```python
from build123d import *

# Parameters (mm, degrees)
BOSS_EXTRUDE1_DEPTH     = 21
SKETCH5_W               = 6.2
SKETCH5_H               = 6.2
CUT_EXTRUDE1_DEPTH      = 4
CUT_EXTRUDE2_DEPTH      = 28.364438602
CUT_EXTRUDE2_DEPTH_BACK = 28.364438602
SKETCH9_W               = 24.284850455
SKETCH9_H               = 22.464844075
CUT_EXTRUDE3_DEPTH      = 2.5


with BuildPart() as part:
    # Sketch3 → Boss-Extrude1 (new body)
    with BuildSketch(Plane(origin=(0, 0, 0), x_dir=(0, 0, -1), z_dir=(1, 0, 0))):
        with BuildLine():
            Line((-12.75, -9.5), (12.75, -9.5))
            ThreePointArc((12.75, -9.5), (14.164213562, -8.914213562), (14.75, -7.5))
            Line((14.75, -7.5), (14.75, 7.5))
            ThreePointArc((14.75, 7.5), (14.164213562, 8.914213562), (12.75, 9.5))
            Line((12.75, 9.5), (-12.75, 9.5))
            ThreePointArc((-12.75, 9.5), (-14.164213562, 8.914213562), (-14.75, 7.5))
            Line((-14.75, 7.5), (-14.75, -7.5))
            ThreePointArc((-14.75, -7.5), (-14.164213562, -8.914213562), (-12.75, -9.5))
        make_face()
    extrude(amount=BOSS_EXTRUDE1_DEPTH)

    # Sketch5 → Cut-Extrude1 (cut)
    with BuildSketch(Plane(origin=(0, 9.5, 0), x_dir=(1, 0, 0), z_dir=(0, 1, 0))):
        with Locations((3.1, 0)):
            Rectangle(SKETCH5_W, SKETCH5_H)
    extrude(amount=-CUT_EXTRUDE1_DEPTH, mode=Mode.SUBTRACT)

    # Sketch7 → Cut-Extrude2 (cut, two sides: drawn at the far end of the back side and taken through both)
    with BuildSketch(Plane.ZY.offset(-CUT_EXTRUDE2_DEPTH_BACK)):
        with BuildLine():
            Line((-11.147623693, -8.072928754), (11.147623693, -8.072928754))
            ThreePointArc((11.147623693, -8.072928754), (12.561837255, -7.487142316), (13.147623693, -6.072928754))
            Line((13.147623693, -6.072928754), (13.147623693, 0.135263404))
            ThreePointArc((13.147623693, 0.135263404), (12.561837255, 1.549476966), (11.147623693, 2.135263404))
            Line((11.147623693, 2.135263404), (-11.147623693, 2.135263404))
            ThreePointArc((-11.147623693, 2.135263404), (-12.561837255, 1.549476966), (-13.147623693, 0.135263404))
            Line((-13.147623693, 0.135263404), (-13.147623693, -6.072928754))
            ThreePointArc((-13.147623693, -6.072928754), (-12.561837255, -7.487142316), (-11.147623693, -8.072928754))
        make_face()
    extrude(amount=CUT_EXTRUDE2_DEPTH + CUT_EXTRUDE2_DEPTH_BACK, mode=Mode.SUBTRACT)

    # Sketch9 → Cut-Extrude3 (cut)
    with BuildSketch(Plane(origin=(0, 9.5, 0), x_dir=(1, 0, 0), z_dir=(0, 1, 0))):
        with Locations((12.142425228, 0.007615305)):
            Rectangle(SKETCH9_W, SKETCH9_H)
    extrude(amount=-CUT_EXTRUDE3_DEPTH, mode=Mode.SUBTRACT)


solid = part.part
```
Geometry: final body of the model. Coordinates: model frame, mm. A direction names the side the tool comes from. Round coordinates to 2 decimals unless told otherwise and drop trailing zeros. Order: outer loops, then holes, each group sorted by start corner. A loop starts at its lowest first (then second) coordinate and runs counter-clockwise, first axis right, second up. Notation, with made-up numbers: (-9.5, 71) -> (6.5, 71) arc R30 ccw to (6.5, 94) -> close; hole circle Ø11 at (15.5, 49). An arc over 180 degrees is marked (long way). Use one line per item in the form item = value.
(1) Ray query, probe 1 along Z at (x, y) = (10.5, -5.25); probe 2 along Y at (x, z) = (2.5, -1.5); probe 3 along Y at (x, z) = (8, 3). Return the intervals inside material, ascending. Write a range as [from, to].
Results list:
probe_1 = [-14.75, -13.15], [13.15, 14.75]
probe_2 = [-9.5, -8.07], [2.14, 5.5]
probe_3 = [-9.5, -8.07], [2.14, 7]
(2) Section D-D on z = 1. Return loops of the section in (x, y), and give its area (3 significant figures).
Results list:
outline = (0, -9.5) -> (21, -9.5) -> (21, -8.07) -> (0, -8.07) -> close; (0, 2.14) -> (21, 2.14) -> (21, 7) -> (6.2, 7) -> (6.2, 5.5) -> (0, 5.5) -> close
area = 123 mm^2
(3) Draft query along Z for faces 6 (the face through (11, -3, -13.148)), 7 (the face through (10.35, -8.93, -14.15)), 8 (the face through (10, 9.5, -12)), 9 (the face through (10.65, 1.56, -12.55)). Return one class per face: pulls with the +Z half, pulls with the -Z half, needs draft (parallel to the pull), parting line crosses it, or undercut.
Results list:
face_6 = undercut
face_7 = pulls with the -Z half
face_8 = needs draft
face_9 = undercut
(4) Section B-B on z = 4.25. Return loops of the section in (x, y).
Results list:
outline = (0, -9.5) -> (21, -9.5) -> (21, -8.07) -> (0, -8.07) -> close; (0, 2.14) -> (21, 2.14) -> (21, 7) -> (0, 7) -> close
(5) Section C-C on x = 18.25. Return loops of the section in (y, z), and give its area (3 significant figures).
Results list:
outline = (-9.5, -12.75) arc R2 ccw to (-7.5, -14.75) -> (7.5, -14.75) arc R2 ccw to (9.5, -12.75) -> (9.5, -11.24) -> (7, -11.24) -> (7, 11.22) -> (9.5, 11.22) -> (9.5, 12.75) arc R2 ccw to (7.5, 14.75) -> (-7.5, 14.75) arc R2 ccw to (-9.5, 12.75) -> close; hole (-8.07, -11.15) arc R2 ccw to (-6.07, -13.15) -> (0.14, -13.15) arc R2 ccw to (2.14, -11.15) -> (2.14, 11.15) arc R2 ccw to (0.14, 13.15) -> (-6.07, 13.15) arc R2 ccw to (-8.07, 11.15) -> close
area = 236 mm^2
(6) First-contact query: pin 1 Ø1.5 at (x, z) = (17.5, -2) entering from +Y; pin 2 Ø2 at (x, y) = (8.5, 8.5) entering from -Z; pin 3 Ø0.8 at (x, y) = (11, 9) entering from +Z. Flat tips, straight axial feed; report the tip coordinate or a pass-through.
Results list:
pin_1 = 7
pin_2 = -14.75
pin_3 = 14.42
(7) Section A-A on y = -2. Return loops of the section in (x, z).
Results list:
outline = (0, -14.75) -> (21, -14.75) -> (21, -13.15) -> (0, -13.15) -> close; (0, 13.15) -> (21, 13.15) -> (21, 14.75) -> (0, 14.75) -> close
(8) Access query for faces 1 (the face through (10, 8, -11.24)), 2 (the face through (3, 6, -3.1)), 3 (the face through (10, 9.5, 12)), 4 (the face through (21, 4, 0)), 5 (the face through (10.65, -7.5, 12.55)). Directions: +Z, -Z, +X, -X, +Y, -Y. A direction counts if a zero-diameter tool reaches every point of the face in a straight line with its end or side. Return the directions, or none.
Results list:
face_1 = +X, -X, +Y
face_2 = -X, +Y
face_3 = +Z, -Z, +X, -X, +Y
face_4 = +Z, -Z, +X, +Y, -Y
face_5 = +X, -X
